Answer from the drawing. Dimensions are ordinates in mm from the lowest x, y and z of the part. Give positions to 0.01 mm unless a question says otherwise; leave off trailing zeros. Write each question's results on one line, items separated by ' | '. Start each with the question number.
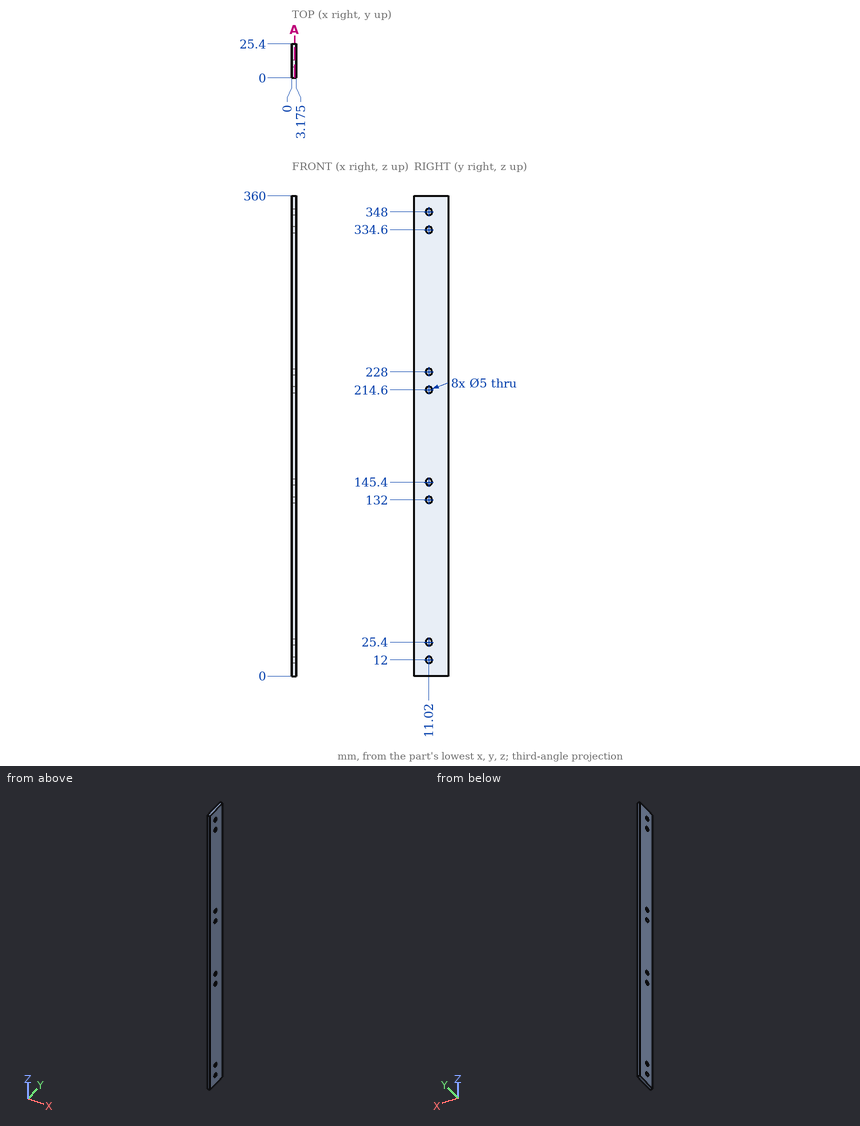
Item 1: Given P1, Ø4, axis at y = 11.02, z = 12, coming from the -X side, flat-ended and moving along its own axis, determine where the tip first touches the part or whether it passes through.
Item 2: Section A-A, the plane x = 2.1 is taken. Give the number of separate pieces and of enclosed holes in the cut face, then the cut area to 3 significant figures.
Item 3: Straight lines are drawn through the part: line 1 (Y direction, x = 2.55, z = 335); line 2 (Y direction, x = 2.75, z = 214.5). For each, find the intervals that lie inside material, in ascending order.
Worked out:
1) P1: passes through
2) separate pieces: 1 | enclosed holes: 8 | area: 8,990 mm²
3) line 1: y = 0 to 8.55, 13.49 to 25.4 | line 2: y = 0 to 8.52, 13.52 to 25.4
